Print and shaded views of the part. All mm, measured from the part's lowest x, y and z. A direction names the side the tool comes from. Give positions to 0.01 mm unless a question says otherwise; leave off trailing zeros. Put each result on its own line as item: value. Start each with the question number.
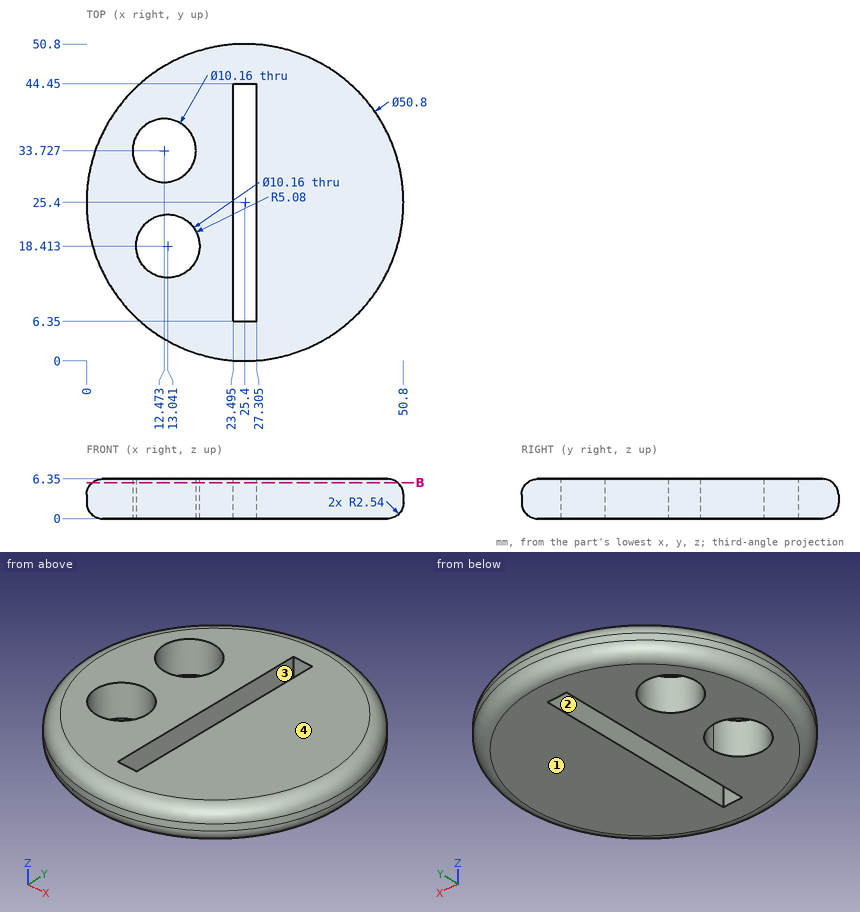
1) Band-saw the part on B-B on z = 5.75. State how many separate pieces and enclosed holes the cut face has, then the cut area to 3 significant figures.
2) Which spindle directions (+Z, -Z, +X, -X, +Y, -Y) get a long thin tool onto all of the face, cutting with end or side? Do the marked faces 3 and 4. Say none if no direction does.
3) Wall check: L1, parallel to Y at x = 8.5, z = 3.5 (1 decimal); L2, parallel to Y at x = 16, z = 5 (1 decimal); L3, parallel to X at y = 23, z = 6 (1 decimal). Give the ranges that are in metal, low to high.
4) Mould opens along X. For the marked faces 1 and 2 say: +X half, -X half, draft (parallel to the pull), parting line (faces both ways), or undercut.
5) Pin check, flat tips, straight feed: pin 1 Ø1 at (x, y) = (6, 9) entering from +Z; pin 2 Ø1 at (y, z) = (43.5, 2.5) entering from +X (1 decimal); pin 3 Ø1.9 at (y, z) = (25.5, 4.5) entering from +X; pin 4 Ø1.9 at (x, z) = (24.5, 2.5) entering from -Y. Stop position of each tip, or through.
Evaluation:
1. separate pieces: 1
1. enclosed holes: 3
1. area: 1,580 mm2
2. face 3: +Z, -Z
2. face 4: +Z, +X, -X, +Y, -Y
3. L1: 6.4 to 16.1, 20.7 to 30.6, 36.9 to 44.4
3. L2: 2.1 to 14.3, 22.5 to 30.1, 37.4 to 48.7
3. L3: 1.4 to 10.9, 15.2 to 23.5, 27.3 to 49.4
4. face 1: draft
4. face 2: undercut
5. pin 1: z = 5.32
5. pin 2: x = 43.7
5. pin 3: x = 50.8
5. pin 4: y = 0
